Source: CAD feature listing. Evaluate the final solid. Frame: model axes, mm. A direction names the side the tool comes from. Round coordinates to 2 decimals unless told otherwise and drop trailing zeros. Order: outer loops, then holes, each group sorted by start corner. A loop starts at its lowest first (then second) coordinate and runs counter-clockwise, first axis right, second up. Notation, with made-up numbers: M 88,87.5 L 137,87.5 A31 cw 137,112.5 Z; hole C 31,76.25 d11. An arc over 180 degrees is marked long. Answer as CSV lines item,"result". Start each with the question number.
Item 1: Line query: line 1 (Y direction, x = -11.65, z = 10); line 2 (X direction, y = -5.75, z = 3); line 3 (Y direction, x = -12, z = 5.75). Output: solid intervals per line, ascending. Write a range as [from, to].
Item 2: Section query B-B on y = 0. Return the cut outline in (x, z), plus the area to 3 significant figures.
Item 3: Section query C-C on x = -11.5. Return the cut outline in (y, z), plus the area to 3 significant figures.
Item 4: Pull-direction query (Z, two-part tool) for faces 5 (the face through (11.78, 1.5, 5.23)), 6 (the face through (11.78, 0.16, 17.5)), 7 (the face through (-12, -7.5, 6)); classes: +Z half, -Z half, draft (parallel to the pull), parting line (faces both ways), or undercut.
Item 5: Section query A-A on z = 3.75. Return the cut outline in (x, y), plus the area to 3 significant figures.
Item 6: Set-up query: faces 1 (the face through (12, 7.5, 6)), 2 (the face through (0, 0, 0)), 3 (the face through (-9.75, 2, 5)), 4 (the face through (12, -7.5, 6)). Return all of +Z, -Z, +X, -X, +Y, -Y with unobstructed straight access to the full face (end or side cutting, diameter ignored); none if empty.
Item 7: First-contact query: P1, Ø1.2, axis at x = -12, z = 5.5, coming from the +Y side; P2, Ø5, axis at x = -4.5, y = 10, coming from the +Z side; P3, Ø4.5, axis at x = 12.5, z = 8, coming from the -Y side. Flat tips, straight axial feed; report the tip coordinate or a pass-through.
Item 8: Section query D-D on z = 7.75. Return the cut outline in (x, y), plus the area to 3 significant figures.
from build123d import *

# Parameters (mm, degrees)
SKETCH1_W               = 27.5
SKETCH1_H               = 27.5
BOSS_EXTRUDE1_DEPTH     = 2.5
SKETCH2_R               = 5
BOSS_EXTRUDE2_DEPTH     = 27.5
CUT_EXTRUDE1_DEPTH      = 9.75
CUT_EXTRUDE1_DEPTH_BACK = 9.75
SKETCH3_W               = 27.5
SKETCH3_H               = 15.762918275


with BuildPart() as part:
    # Sketch1 → Boss-Extrude1 (new body)
    with BuildSketch(Plane(origin=(0, 0, 0), x_dir=(0, 1, 0), z_dir=(0, 0, 1))):
        Rectangle(SKETCH1_W, SKETCH1_H)
    extrude(amount=BOSS_EXTRUDE1_DEPTH)

    # Sketch2 → Boss-Extrude2 (add)
    with BuildSketch(Plane.YZ.offset(13.75)):
        with BuildLine():
            Line((-7.5, 2.5), (7.5, 2.5))
            Line((7.5, 2.5), (7.5, 10))
            ThreePointArc((7.5, 10), (0, 17.5), (-7.5, 10))
            Line((-7.5, 10), (-7.5, 2.5))
        make_face()
        with Locations(Location((0, 10, 0), (0, 0, 270))):
            Circle(SKETCH2_R, mode=Mode.SUBTRACT)
    extrude(amount=-BOSS_EXTRUDE2_DEPTH)

    # Sketch3 → Cut-Extrude1 (cut, two sides: drawn at the far end of the back side and taken through both)
    with BuildSketch(Plane.YZ.offset(-CUT_EXTRUDE1_DEPTH_BACK)):
        with Locations((0, 10.381459138)):
            Rectangle(SKETCH3_W, SKETCH3_H)
    extrude(amount=CUT_EXTRUDE1_DEPTH + CUT_EXTRUDE1_DEPTH_BACK, mode=Mode.SUBTRACT)


solid = part.part
Results:
1,line 1,"[-7.5, -5], [5, 7.5]"
1,line 2,"[-13.75, -9.75], [9.75, 13.75]"
1,line 3,"[-7.5, -2.63], [2.63, 7.5]"
2,outline,"M -13.75,0 L 13.75,0 L 13.75,5 L 9.75,5 L 9.75,2.5 L -9.75,2.5 L -9.75,5 L -13.75,5 Z; M -13.75,15 L -9.75,15 L -9.75,17.5 L -13.75,17.5 Z; M 9.75,15 L 13.75,15 L 13.75,17.5 L 9.75,17.5 Z"
2,area,"109 mm^2"
3,outline,"M -13.75,0 L 13.75,0 L 13.75,2.5 L 7.5,2.5 L 7.5,10 A7.5 ccw -7.5,10 L -7.5,2.5 L -13.75,2.5 Z; hole C 0,10 d10"
3,area,"191 mm^2"
4,face 5,"undercut"
4,face 6,"+Z half"
4,face 7,"draft"
5,outline,"M -13.75,-7.5 L -9.75,-7.5 L -9.75,7.5 L -13.75,7.5 Z; M 9.75,-7.5 L 13.75,-7.5 L 13.75,7.5 L 9.75,7.5 Z"
5,area,"120 mm^2"
6,face 1,"+Z, +X, -X, +Y"
6,face 2,"-Z, +X, -X, +Y, -Y"
6,face 3,"+Z, +Y, -Y"
6,face 4,"+Z, +X, -X, -Y"
7,P1,"y = 7.5"
7,P2,"z = 2.5"
7,P3,"y = -7.5"
8,outline,"M -13.75,-7.5 L -9.75,-7.5 L -9.75,-4.47 L -13.75,-4.47 Z; M -13.75,4.47 L -9.75,4.47 L -9.75,7.5 L -13.75,7.5 Z; M 9.75,-7.5 L 13.75,-7.5 L 13.75,-4.47 L 9.75,-4.47 Z; M 9.75,4.47 L 13.75,4.47 L 13.75,7.5 L 9.75,7.5 Z"
8,area,"48.6 mm^2"
